```python
from build123d import *

# Parameters (mm, degrees)
SKETCH2_W                    = 110
SKETCH2_H                    = 80
BOSS_EXTRUDE1_DEPTH          = 23
SKETCH3_R                    = 9.1
THREAD_EXTRUDE_DEPTH         = 45
SKETCH5_R                    = 11.85
NUT_EXTRUDE_DEPTH            = 17
SKETCH6_R                    = 8.4
MINOR_DIANETER_EXTRUDE_DEPTH = 64
CABLE_EXTRUDE_DEPTH          = 138.945641468


with BuildPart() as part:
    # Sketch2 → Boss-Extrude1 (new body)
    with BuildSketch(Plane.XY):
        with Locations((55, 40)):
            Rectangle(SKETCH2_W, SKETCH2_H)
    extrude(amount=BOSS_EXTRUDE1_DEPTH)

    # Sketch3 → Thread extrude (cut)
    with BuildSketch(Plane(origin=(0, 80, 0), x_dir=(1, 0, 0), z_dir=(0, 1, 0))):
        with Locations((20, -7)):
            Circle(SKETCH3_R)
        with Locations((90, -7)):
            Circle(SKETCH3_R)
    extrude(amount=-THREAD_EXTRUDE_DEPTH, mode=Mode.SUBTRACT)

    # Sketch5 → Nut extrude (cut)
    with BuildSketch(Plane(origin=(0, 80, 0), x_dir=(1, 0, 0), z_dir=(0, 1, 0))):
        with Locations((20, -7)):
            Circle(SKETCH5_R)
        with Locations((90, -7)):
            Circle(SKETCH5_R)
    extrude(amount=-NUT_EXTRUDE_DEPTH, mode=Mode.SUBTRACT)

    # Sketch6 → minor dianeter extrude (cut)
    with BuildSketch(Plane(origin=(0, 80, 0), x_dir=(1, 0, 0), z_dir=(0, 1, 0))):
        with Locations((20, -7)):
            Circle(SKETCH6_R)
        with Locations((90, -7)):
            Circle(SKETCH6_R)
    extrude(amount=-MINOR_DIANETER_EXTRUDE_DEPTH, mode=Mode.SUBTRACT)

    # Sketch4 → Cable extrude (cut, through all)
    with BuildSketch(Plane(origin=(0, 80, 0), x_dir=(1, 0, 0), z_dir=(0, 1, 0))):
        with BuildLine():
            Line((17, -7), (17, 0))
            Line((17, 0), (23, 0))
            Line((23, 0), (23, -7))
            ThreePointArc((23, -7), (20, -10), (17, -7))
        make_face()
        with BuildLine():
            Line((87, -7), (87, 0))
            Line((87, 0), (93, 0))
            Line((93, 0), (93, -7))
            ThreePointArc((93, -7), (90, -10), (87, -7))
        make_face()
    extrude(amount=-CABLE_EXTRUDE_DEPTH, mode=Mode.SUBTRACT)


solid = part.part
```
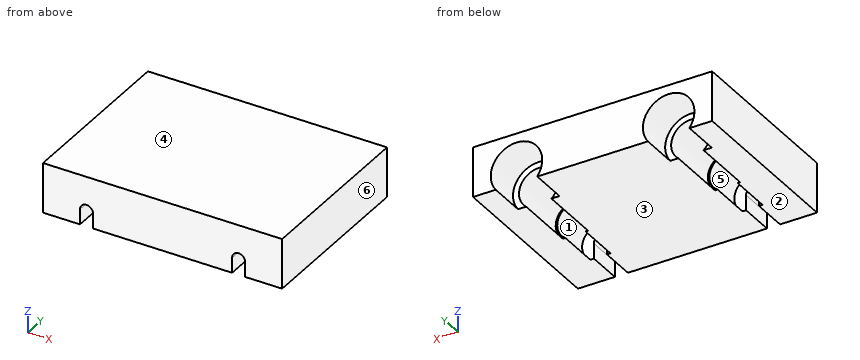
Design review of the part built by this model. Coordinates are the model's own, in mm. Face numbers are marked on the shaded views. A direction names the side the tool comes from. Round coordinates to 2 decimals unless told otherwise and drop trailing zeros. Order: outer loops, then holes, each group sorted by start corner. A loop starts at its lowest first (then second) coordinate and runs counter-clockwise, first axis right, second up. Notation, with made-up numbers: M 22,26.5 L 59,26.5 A26 ccw 59,48.5 Z; hole C 37.5,-29.5 d4. An arc over 180 degrees is marked long. Put each result on its own line as item: value.
Q1. Consider section C-C (z = 13.25). State the section outline as (x, y) points.
Reported:
outline: M 0,0 L 110,0 L 110,80 L 100.07,80 L 100.07,63 L 96.61,63 L 96.61,35 L 95.61,35 L 95.61,16 L 84.39,16 L 84.39,35 L 83.39,35 L 83.39,63 L 79.93,63 L 79.93,80 L 30.07,80 L 30.07,63 L 26.61,63 L 26.61,35 L 25.61,35 L 25.61,16 L 14.39,16 L 14.39,35 L 13.39,35 L 13.39,63 L 9.93,63 L 9.93,80 L 0,80 Z
Q2. Consider section D-D (y = 42). State the section outline as (x, z) points, and give its area (3 significant figures).
Reported:
outline: M 0,0 L 14.19,0 A9.1 cw long 25.81,0 L 84.19,0 A9.1 cw long 95.81,0 L 110,0 L 110,23 L 0,23 Z
area: 2,040 mm²
Q3. Consider section B-B (y = 7.5). State the section outline as (x, z) points, and give its area (3 significant figures).
Reported:
outline: M 0,0 L 17,0 L 17,7 A3 cw 23,7 L 23,0 L 87,0 L 87,7 A3 cw 93,7 L 93,0 L 110,0 L 110,23 L 0,23 Z
area: 2,420 mm²
Q4. Insertion check: pin 1 Ø9.5 at (x, z) = (19.5, 12.5) entering from +Y; pin 2 Ø4.5 at (x, z) = (88, 11) entering from +Y. Each pin has a flat end and moves straight along its axis. Give the tip position at first contact, or say it passes through.
Reported:
pin 1: y = 63
pin 2: y = 16
Q5. Draft analysis for pull direction Z (two halves, no side actions). For the marked faces 3, 4, 5 and 6, state which applies: released by +Z, released by -Z, zero draft, split by the parting line, or undercut.
Reported:
face 3: released by -Z
face 4: released by +Z
face 5: undercut
face 6: zero draft
Q6. Machinability: for the marked faces 1 and 2, which of the approach directions +Z, -Z, +X, -X, +Y, -Y give a long, thin tool a straight path to every point of the face, cutting with its end or side? Answer none if there is none.
Reported:
face 1: +Y
face 2: -Z, +X, -X, +Y, -Y
Q7. To check wall thickness, follow line 1 (X direction, y = 53.5, z = 3.5); line 2 (X direction, y = 54.5, z = 7); line 3 (Z direction, x = 90, y = 72.5). State the ranges of each line that lie inside material, in increasing order.
Reported:
line 1: 0 to 11.6, 28.4 to 81.6, 98.4 to 110
line 2: 0 to 10.9, 29.1 to 80.9, 99.1 to 110
line 3: 18.85 to 23
Q8. Consider section A-A (x = 90). State the section outline as (y, z) points, and give its area (3 significant figures).
Reported:
outline: M 0,10 L 16,10 L 16,15.4 L 35,15.4 L 35,16.1 L 63,16.1 L 63,18.85 L 80,18.85 L 80,23 L 0,23 Z
area: 616 mm²
